Model file for the job. Use its own axes, mm. Give positions to 0.01 mm unless a question says otherwise; leave off trailing zeros. Write each loop counter-clockwise with the first axis right and the second up, starting at its lowest first coordinate (ties: lowest second). Pieces come first, ordered by that corner, then holes. Notation, with made-up numbers: (88.5, 57) - (118.5, 57) arc R8 cw to (118.5, 68) - close; hole circle Ø7 at (-0.5, 55). An arc over 180 degrees is marked (long way). Use a Markdown table: item, result. Add a question column.
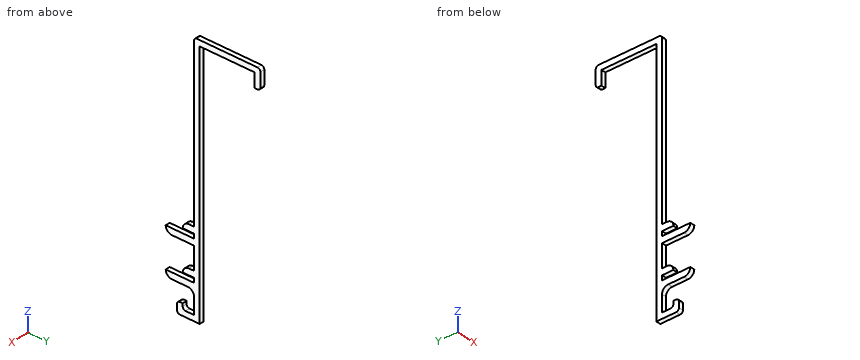
```python
from build123d import *

# Parameters (mm, degrees)
F1_DEPTH = 8
F2_R     = 10.99999
F3_R     = 10.99999
F4_R     = 10.99999
F5_R     = 10.99999
F6_R     = 5
F7_R     = 5


# Not quite as in the source:
# - a fillet or chamfer is up to 0.001 mm smaller than in the source, because OpenCascade refuses the exact size


with BuildPart() as f1:
    # F0 (on Right) → F1 (new body)
    with BuildSketch(Plane.YZ):
        Polygon((115.3961805266, 292.9259983301), (-1.6038194734, 292.9259983301), (-1.6038194734, -7.0740016699), (-21.6038194734, -7.0740016699), (-21.6038194734, -18.0740016699), (-1.6038194734, -18.0740016699), (-1.6038194734, -26.0740016699), (-51.6038194734, -26.0740016699), (-51.6038194734, -37.0740016699), (-1.6038194734, -37.0740016699), (-1.6038194734, -77.0740016699), (-21.6038194734, -77.0740016699), (-21.6038194734, -88.0740016699), (-1.6038194734, -88.0740016699), (-1.6038194734, -96.0740016699), (-51.6038194734, -96.0740016699), (-51.6038194734, -107.0740016699), (-1.6038194734, -107.0740016699), (-1.6038194734, -147.0740016699), (-21.6038194734, -147.0740016699), (-21.6038194734, -137.0740016699), (-31.6038194734, -137.0740016699), (-31.6038194734, -157.0740016699), (8.3961805266, -157.0740016699), (8.3961805266, 282.9259983301), (105.3961805266, 282.9259983301), (105.3961805266, 257.9259983301), (115.3961805266, 257.9259983301), align=None)
    extrude(amount=-F1_DEPTH)

    # F2 (radius 11 in the source; OpenCascade refuses exactly that, so slightly less here)
    f2_edges = [f1.edges().sort_by_distance(p)[0] for p in [
        (-4, -51.603819, -37.074002),
    ]]
    fillet(f2_edges, radius=F2_R)

    # F3 (radius 11 in the source; OpenCascade refuses exactly that, so slightly less here)
    f3_edges = [f1.edges().sort_by_distance(p)[0] for p in [
        (-4, -21.603819, -7.074002),
    ]]
    fillet(f3_edges, radius=F3_R)

    # F4 (radius 11 in the source; OpenCascade refuses exactly that, so slightly less here)
    f4_edges = [f1.edges().sort_by_distance(p)[0] for p in [
        (-4, -21.603819, -77.074002),
    ]]
    fillet(f4_edges, radius=F4_R)

    # F5 (radius 11 in the source; OpenCascade refuses exactly that, so slightly less here)
    f5_edges = [f1.edges().sort_by_distance(p)[0] for p in [
        (-4, -51.603819, -107.074002),
        (-4, -1.603819, -107.074002),
    ]]
    fillet(f5_edges, radius=F5_R)

    # F6
    f6_edges = [f1.edges().sort_by_distance(p)[0] for p in [
        (-4, -31.603819, -137.074002),
        (-4, -31.603819, -157.074002),
        (-4, -21.603819, -147.074002),
    ]]
    fillet(f6_edges, radius=F6_R)

    # F7
    f7_edges = [f1.edges().sort_by_distance(p)[0] for p in [
        (-4, -1.603819, 292.925998),
        (-4, 115.396181, 292.925998),
        (-4, 115.396181, 257.925998),
    ]]
    fillet(f7_edges, radius=F7_R)


solid = f1.part
```
(1) Flat gauge pins, fed straight in: pin 1 (2.5 mm diameter, centred on x = -2, y = -7.5, fed in from +Z); pin 2 (4 mm diameter, centred on x = -3.5, z = -145, fed in from -Y); pin 3 (1.5 mm diameter, centred on x = -5, y = -25, fed in from +Z). Where does each tip first touch, or does it go through?
(2) Band-saw the part on A-A (z = 86.5). Write the cut outline in (x, y).
(3) Band-saw the part on B-B (y = 51). Write the cut outline in (x, z), then the cut area to 3 significant figures.
(4) Probe probe 1 along Z at (x, y) = (-4.25, -22); probe 2 along Z at (x, y) = (-4, -30.5); probe 3 along Z at (x, y) = (-2, -3). List the from-to ranges inside material, lowest first. Write a range as [from, to].
Model answer:
| question | item | result |
|---|---|---|
| 1 | pin 1 | stops at z = -7.07 |
| 1 | pin 2 | stops at y = -31.6 |
| 1 | pin 3 | stops at z = -26.07 |
| 2 | outline | (-8, -1.6) - (0, -1.6) - (0, 8.4) - (-8, 8.4) - close |
| 3 | outline | (-8, 282.93) - (0, 282.93) - (0, 292.93) - (-8, 292.93) - close |
| 3 | area | 80.0 mm^2 |
| 4 | probe 1 | z = [-157.07, -137.07], [-107.07, -96.07], [-37.07, -26.07] |
| 4 | probe 2 | z = [-155.21, -138.94], [-107.07, -96.07], [-37.07, -26.07] |
| 4 | probe 3 | z = [-157.07, -147.07], [-112.71, -96.07], [-88.07, -77.07], [-37.07, -26.07], [-18.07, -7.07] |
